Part print with two shaded views. Sizes in mm from the minimum x, y, z corner. Round coordinates to 2 decimals unless told otherwise and drop trailing zeros. Order: outer loops, then holes, each group sorted by start corner. A loop starts at its lowest first (then second) coordinate and runs counter-clockwise, first axis right, second up. Notation, with made-up numbers: (-28, 38.25) -> (-1, 38.25) arc R9 ccw to (-1, 42.25) -> close; hole circle Ø6 at (83, 23.25). An arc over 180 degrees is marked (long way). Use a Markdown table: item, result. Add a question column.
Item 1: Pin check, flat tips, straight feed: pin 1 (3 mm diameter, centred on y = 23, z = 22, fed in from +X); pin 2 (10 mm diameter, centred on y = 33.5, z = 23.5, fed in from -X). Stop position of each tip, or through.
Item 2: Slice it at B-B, the plane z = 29.5. Give the cut face in (x, y).
Item 3: Probe L1, parallel to X at y = 26.5, z = 14.5; L2, parallel to X at y = 3, z = 5; L3, parallel to Z at x = 44.5, y = 6.5. List the from-to ranges inside material, lowest first.
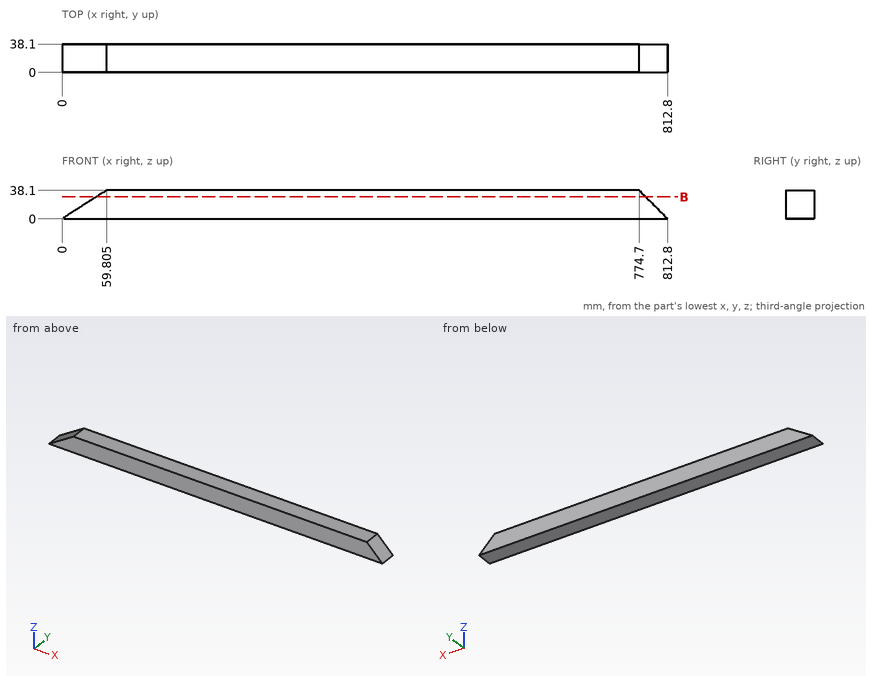
Check sheet entries:
| question | item | result |
|---|---|---|
| 1 | pin 1 | x = 792.3 |
| 1 | pin 2 | x = 29.04 |
| 2 | outline | (46.31, 0) -> (783.3, 0) -> (783.3, 38.1) -> (46.31, 38.1) -> close |
| 3 | L1 | 22.76 to 798.3 |
| 3 | L2 | 7.85 to 807.8 |
| 3 | L3 | 0 to 28.35 |
